Study the drawing (mm; zero at the part's minimum x, y, z) and answer. Coordinates: 2 decimals unless noted, no trailing zeros. Write each loop counter-clockwise with the first axis right and the second up, starting at its lowest first coordinate (ties: lowest second). Pieces come first, ordered by that corner, then holes. Notation, with made-up numbers: M -15,59.25 L 35,59.25 A33 cw 35,98.25 Z; hole C 33.5,86.25 d9. An arc over 180 degrees is marked long. Answer as CSV lines item,"result". Start each with the question number.
(1) A cutting plane is placed at A-A on y = 0.8. Give the vertices of the cut face in (x, z) (1 decimal), then the cut area to 3 significant figures.
(2) Find the intervals of material crossed by L1, parallel to X at y = 2.6, z = 4.5 (1 decimal); L2, parallel to X at y = 1.9, z = 0.75 (1 decimal); L3, parallel to Z at x = 0.5, y = 2.9 (1 decimal), in increasing order. Write a range as [from, to].
(3) A cutting plane is placed at B-B on x = 11. Give the vertices of the cut face in (y, z).
(4) A cutting plane is placed at C-C on z = 2.5. Give the vertices of the cut face in (x, y) (1 decimal), then the cut area to 3 significant figures.
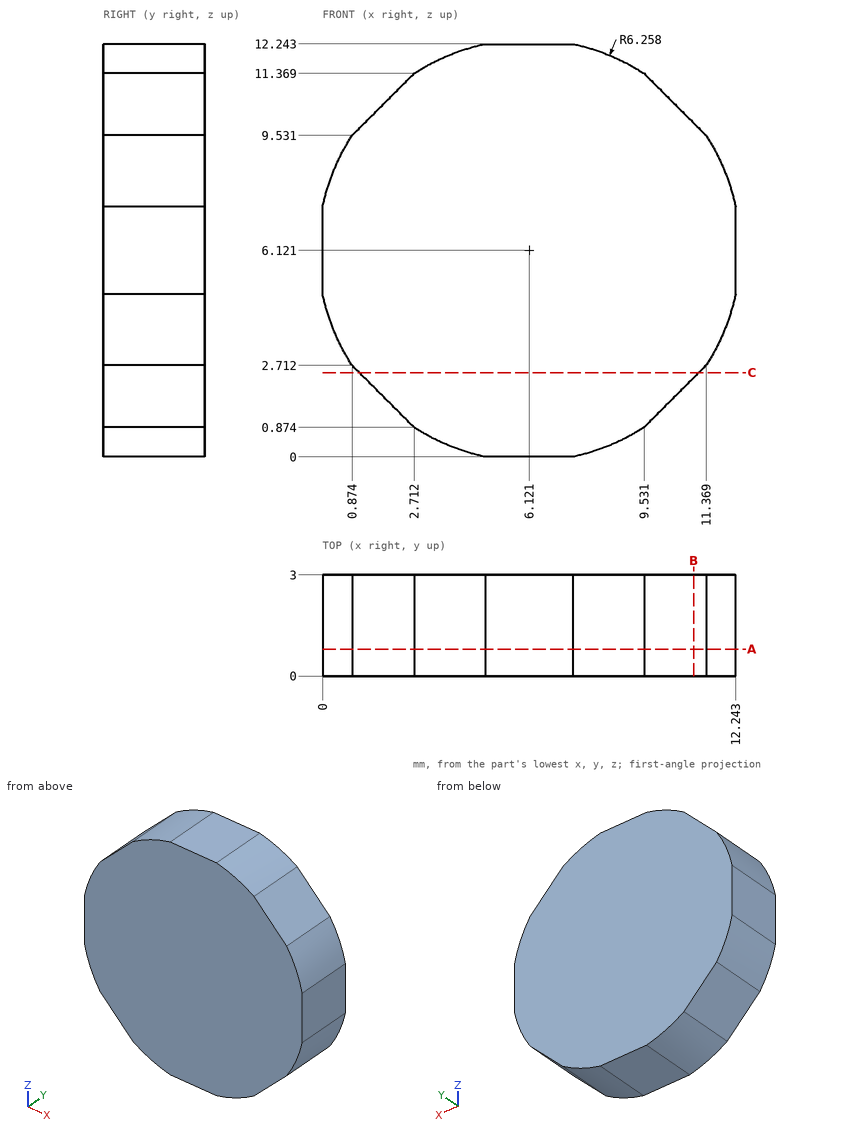
Here are the results:
1,outline,"M 0,4.8 A6.3 ccw 0.9,2.7 L 2.7,0.9 A6.3 ccw 4.8,0 L 7.4,0 A6.3 ccw 9.5,0.9 L 11.4,2.7 A6.3 ccw 12.2,4.8 L 12.2,7.4 A6.3 ccw 11.4,9.5 L 9.5,11.4 A6.3 ccw 7.4,12.2 L 4.8,12.2 A6.3 ccw 2.7,11.4 L 0.9,9.5 A6.3 ccw 0,7.4 Z"
1,area,"121 mm^2"
2,L1,"x = [0.1, 12.2]"
2,L2,"x = [2.9, 9.3]"
2,L3,"z = [3.4, 8.9]"
3,outline,"M 0,2.34 L 3,2.34 L 3,9.9 L 0,9.9 Z"
4,outline,"M 1.1,0 L 11.2,0 L 11.2,3 L 1.1,3 Z"
4,area,"30.2 mm^2"
